Can you work these out from the model? Positions are in its coordinate system, mm. Face numbers are marked on the shaded views. A direction names the side the tool comes from. Round coordinates to 2 decimals unless told otherwise and drop trailing zeros. Order: outer loops, then holes, each group sorted by start corner. A loop starts at its lowest first (then second) coordinate and runs counter-clockwise, first axis right, second up.
Q1. If we section it at A-A (x = 84.5): Please give me the cut outline in (y, z).
Q2. We'd pull the mould along Z, two halves only. Please class the marked faces 1, 2, 3 and 4: pulls with the +Z half, pulls with the -Z half, needs draft (parallel to the pull), parting line crosses it, or undercut.
Q3. If I drill on line 1 (X direction, y = 51, z = 2.25); line 2 (X direction, y = -8, z = 51); line 3 (Z direction, x = 42, y = -38), over which ranges is the centre line in solid material (lowest first)?
Q4. Will these pins go through, and if not, where does the flat tip stop? P1, Ø5.5, axis at x = 28.5, y = -51, coming from the -Z side; P2, Ø7, axis at x = 47, y = 53.5, coming from the -Z side; P3, Ø18.5, axis at x = 61, y = 47.5, coming from the +Z side.
Q5. If we section it at D-D (y = -49): Please give me the cut outline in (x, z).
Q6. If we section it at C-C (x = 55): Please give me the cut outline in (y, z), plus the area to 3 significant figures.
Q7. If we section it at B-B (y = 29): Please give me the cut outline in (x, z), plus the area to 3 significant figures.
Q8. For the marked faces 5, 6 and 7, which set-ups out of +Z, -Z, +X, -X, +Y, -Y let a thin tool reach every point of the face, with its end or its side?
from build123d import *

# Parameters (mm, degrees)
SKETCH_R     = 53.5
PAD_DEPTH    = 134
SKETCH004_R  = 5
PAD002_DEPTH = 20
PAD001_DEPTH = 74
SKETCH002_R  = 4.5
POCKET_DEPTH = 5


with BuildPart() as motorbody:
    # Sketch → Pad (new body)
    with BuildSketch(Plane.YZ):
        Circle(SKETCH_R)
    extrude(amount=PAD_DEPTH)

    # Sketch004 (on Face2 of Pad) → Pad002 (join)
    with BuildSketch(Plane(origin=(0, 0, 0), x_dir=(0, 1, 0), z_dir=(-1, 0, 0))):
        Circle(SKETCH004_R)
    extrude(amount=PAD002_DEPTH)


with BuildPart() as motor:
    # Sketch001 → Pad001 (new body)
    with BuildSketch(Plane.YZ):
        with BuildLine():
            ThreePointArc((-26.5, -46.4758001545), (-13.7075652786, -51.7141436566), (0, -53.5))
            Line((0, -53.5), (0, -57.5))
            ThreePointArc((-26.5, -51.0294032887), (-13.6392688752, -55.8589325404), (0, -57.5))
            Line((-26.5, -51.0294032887), (-37, -57))
            Line((-37, -57), (-60, -57))
            Line((-60, -57), (-60, -53))
            Line((-60, -53), (-37, -53))
            Line((-26.5, -46.4758001545), (-37, -53))
        make_face()
    pad001 = extrude(amount=PAD001_DEPTH)

    # Sketch002 (on Face4 of Pad001) → Pocket (cut)
    with BuildSketch(Plane(origin=(0, 0, -53), x_dir=(0, -1, 0), z_dir=(0, 0, 1))):
        with Locations((51, 66)):
            Circle(SKETCH002_R)
        with Locations((51, 10)):
            Circle(SKETCH002_R)
    pocket = extrude(amount=-POCKET_DEPTH, mode=Mode.SUBTRACT)

    # Mirrored: Pad001 across Sketch001 V_Axis
    add(pad001.mirror(Plane(origin=(0, 0, 0), x_dir=(1, 0, 0), z_dir=(0, 1, 0))))

    # Mirrored001: Pocket across Sketch002 V_Axis
    add(pocket.mirror(Plane(origin=(0, 0, -53), x_dir=(0, 0, 1), z_dir=(0, -1, 0))), mode=Mode.SUBTRACT)


with BuildPart() as motor_1:
    # Body001 placement: moved
    add(motor.part.moved(Location((18.5, 0, 0))))

    # Connect: union MotorBody
    add(motorbody.part)


with BuildPart() as motor_2:
    # Connect placement: moved
    add(motor_1.part.moved(Location((0, 0, 57))))


solid = motor_2.part
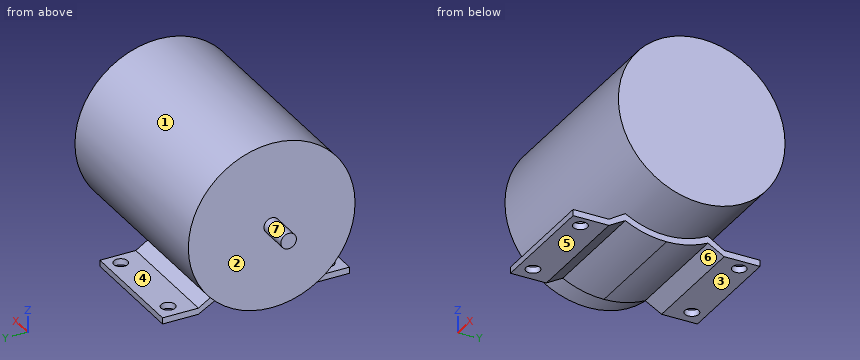
Solution:
1. outline: (-60, 0) - (-55.5, 0) - (-55.5, 4) - (-60, 4) - close; (-46.5, 0) - (-37, 0) - (-26.5, 5.97) arc R57.5 ccw to (26.5, 5.97) - (37, 0) - (46.5, 0) - (46.5, 4) - (37, 4) - (26.5, 10.52) arc R53.5 ccw (long way) to (-26.5, 10.52) - (-37, 4) - (-46.5, 4) - close; (55.5, 0) - (60, 0) - (60, 4) - (55.5, 4) - close
2. face 1: undercut
2. face 2: needs draft
2. face 3: pulls with the -Z half
2. face 4: undercut
3. line 1: x = 18.5 to 24, 33 to 80, 89 to 92.5
3. line 2: x = 0 to 134
3. line 3: z = 0 to 4, 19.34 to 94.66
4. P1: stops at z = 33.89
4. P2: stops at z = 0
4. P3: stops at z = 94.41
5. outline: (0, 35.52) - (134, 35.52) - (134, 78.48) - (0, 78.48) - close; (18.5, 0) - (24.47, 0) - (24.47, 4) - (18.5, 4) - close; (32.53, 0) - (80.47, 0) - (80.47, 4) - (32.53, 4) - close; (88.53, 0) - (92.5, 0) - (92.5, 4) - (88.53, 4) - close
6. outline: (-60, 0) - (-37, 0) - (-26.5, 5.97) arc R57.5 ccw to (26.5, 5.97) - (37, 0) - (60, 0) - (60, 4) - (37, 4) - (26.5, 10.52) arc R53.5 ccw (long way) to (-26.5, 10.52) - (-37, 4) - (-60, 4) - close
6. area: 9,490 mm2
7. outline: (0, 12.04) - (134, 12.04) - (134, 101.96) - (0, 101.96) - close; (18.5, 4.55) - (92.5, 4.55) - (92.5, 8.97) - (18.5, 8.97) - close
7. area: 12,400 mm2
8. face 5: -Z, +X, -X, -Y
8. face 6: -Z, +X, -X
8. face 7: -X
